```python
from build123d import *

# Parameters (mm, degrees)
F0_R     = 30
F1_DEPTH = 90
F2_T     = -2.5
F3_R     = 2.5
F4_R     = 5
F5_R     = 1.24999


# Not quite as in the source:
# - a fillet or chamfer is up to 0.001 mm smaller than in the source, because OpenCascade refuses the exact size


with BuildPart() as f1:
    # F0 (on Top) → F1 (new body)
    with BuildSketch(Plane.XY):
        Circle(F0_R)
    extrude(amount=F1_DEPTH)

    # F2
    f2_openings = [f1.faces().sort_by_distance(p)[0] for p in [
        (0, 0, 90),
    ]]
    offset(amount=F2_T, openings=f2_openings)

    # F3
    f3_edges = [f1.edges().sort_by_distance(p)[0] for p in [
        (-27.5, 0, 2.5),
    ]]
    fillet(f3_edges, radius=F3_R)

    # F4
    f4_edges = [f1.edges().sort_by_distance(p)[0] for p in [
        (-30, 0, 0),
    ]]
    fillet(f4_edges, radius=F4_R)

    # F5 (radius 1.25 in the source; OpenCascade refuses exactly that, so slightly less here)
    f5_edges = [f1.edges().sort_by_distance(p)[0] for p in [
        (-30, 0, 90),
        (-27.5, 0, 90),
    ]]
    fillet(f5_edges, radius=F5_R)


solid = f1.part
```
CAD build for the part. Positions are in the model's coordinates, mm. Coordinates: 2 decimals unless noted, no trailing zeros. Order: outer loops, then holes, each group sorted by start corner. A loop starts at its lowest first (then second) coordinate and runs counter-clockwise, first axis right, second up. Notation, with made-up numbers: (87, 69) - (131, 69) arc R21 ccw to (131, 84) - close; hole circle Ø10 at (-38, -25). An arc over 180 degrees is marked (long way). Use a Markdown table: item, result. Add a question column.
(1) Drill centre lines: line 1 along Y through (x, z) = (0, 35); line 2 along X through (y, z) = (1, 68); line 3 along Z through (x, y) = (-13, 17.5). Where is each one in solid material? Low to high. Write a range as [from, to].
(2) Flat gauge pins, fed straight in: pin 1 (6 mm diameter, centred on x = -8.5, z = 39, fed in from +Y); pin 2 (1.5 mm diameter, centred on x = -23.5, z = 60.5, fed in from -Y); pin 3 (10 mm diameter, centred on y = 16.5, z = 54, fed in from -X). Where does each tip first touch, or does it go through?
(3) Saw through at C-C (z = 57). Give the cut face in (x, y).
(4) Pull direction Y, two halves, no side cores. Call faces 1 (the face through (-5.961, -26.846, 46.289)), 2 (the face through (-29.97, 1.32, 46.29)), 3 (the face through (0, 0, 0)): +Y half, -Y half, draft (parallel to the pull), parting line (faces both ways), or undercut.
Solved:
| question | item | result |
|---|---|---|
| 1 | line 1 | y = [-30, -27.5], [27.5, 30] |
| 1 | line 2 | x = [-29.98, -27.48], [27.48, 29.98] |
| 1 | line 3 | z = [0, 2.5] |
| 2 | pin 1 | stops at y = 29.49 |
| 2 | pin 2 | stops at y = -19.56 |
| 2 | pin 3 | stops at x = -27.71 |
| 3 | outline | circle Ø60 at (0, 0); hole circle Ø55 at (0, 0) |
| 4 | face 1 | undercut |
| 4 | face 2 | parting line |
| 4 | face 3 | draft |
